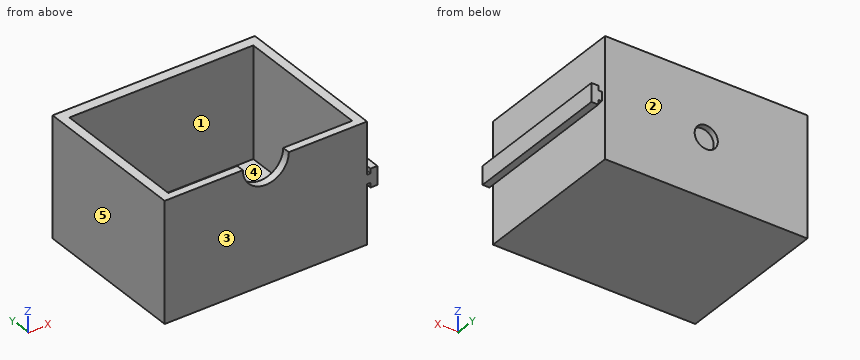
from build123d import *

# Parameters (mm, degrees)
F0_W     = 55.88
F0_H     = 33.02
F1_DEPTH = 43.18
F2_W     = 50.8
F2_H     = 38.1
F3_DEPTH = 30.48
F4_R     = 6.35
F5_DEPTH = 25.4
F6_R     = 3.2
F7_DEPTH = 1.6002
F9_DEPTH = 41.91


with BuildPart() as f1:
    # F0 (on Front) → F1 (new body)
    with BuildSketch(Plane.XZ):
        with Locations((-20.484024, 16.51)):
            Rectangle(F0_W, F0_H)
    extrude(amount=-F1_DEPTH)

    # F2 (on face) → F3 (cut)
    with BuildSketch(Plane.XY.offset(33.02)):
        with Locations((-20.484024, 21.216264)):
            Rectangle(F2_W, F2_H)
    extrude(amount=-F3_DEPTH, mode=Mode.SUBTRACT)

    # F4 (on face) → F5 (cut)
    with BuildSketch(Plane.XZ):
        with Locations((-20.484024, 33.02)):
            Circle(F4_R)
    extrude(amount=-F5_DEPTH, mode=Mode.SUBTRACT)

    # F6 (on face) → F7 (cut)
    with BuildSketch(Plane(origin=(0, 43.18, 0), x_dir=(-1, 0, 0), z_dir=(0, 1, 0))):
        with Locations((20.484024, 16.51)):
            Circle(F6_R)
    extrude(amount=-F7_DEPTH, mode=Mode.SUBTRACT)

    # F8 (on face) → F9 (join)
    with BuildSketch(Plane.XZ):
        Polygon((8.421195, 20.018721), (8.421195, 18.748721), (7.455976, 18.748721), (7.455976, 16.208721), (8.421195, 16.208721), (8.421195, 14.938721), (10.326195, 14.938721), (10.326195, 20.018721), align=None)
    extrude(amount=-F9_DEPTH)


solid = f1.part
The listing builds one solid part. Answer for the finished solid, in the listing's coordinates (mm). Face numbers are marked on the shaded views. A direction names the side the tool comes from. Round coordinates to 2 decimals unless told otherwise and drop trailing zeros. Order: outer loops, then holes, each group sorted by start corner. A loop starts at its lowest first (then second) coordinate and runs counter-clockwise, first axis right, second up. Notation, with made-up numbers: (9.5, -22) - (65.5, -22) arc R25 cw to (65.5, -1) - close; hole circle Ø11 at (-19.75, -21). An arc over 180 degrees is marked (long way). Write item = value, one per line. Start each with the question number.
1) Straight lines are drawn through the part: L1, parallel to Y at x = -9.5, z = 23; L2, parallel to X at y = 23, z = 22.5; L3, parallel to Z at x = -5, y = 22. For each, find the intervals that lie inside material, in ascending order.
2) Given pin 1 (4 mm diameter, centred on x = -20.48, z = 16.51, fed in from +Y); pin 2 (10 mm diameter, centred on x = -21, z = 29.5, fed in from -Y); pin 3 (1.5 mm diameter, centred on x = 9, y = 17.5, fed in from +Z); pin 4 (5 mm diameter, centred on y = 32, z = 11, fed in from +X), each flat-ended and moving along its own axis, determine where each tip first touches the part or whether it passes through.
3) Section D-D, the plane z = 28 is taken. Write down the section's boundary in (x, y), plus the area to 3 significant figures.
4) For the marked faces 1 and 2, determine the directions among +Z, -Z, +X, -X, +Y, -Y from which every point of the face is accessible in a straight line to the end or side of a thin tool.
5) For a pull along X with two mould halves and no side action, classify the marked faces 3, 4 and 5 as released by +X, released by -X, zero draft, split by the parting line, or undercut.
6) Section A-A, the plane z = 8.5 is taken. Write down the section's boundary in (x, y).
7) Section C-C, the plane y = 16 is taken. Write down the section's boundary in (x, z).
8) Section B-B, the plane x = -2 is taken. Write down the section's boundary in (y, z), plus the area to 3 significant figures.
Results list:
q1.L1 = 0 to 2.17, 40.27 to 43.18
q1.L2 = -48.42 to -45.88, 4.92 to 7.46
q1.L3 = 0 to 2.54
q2.pin_1 = 41.58
q2.pin_2 = 0
q2.pin_3 = 20.02
q2.pin_4 = 7.46
q3.outline = (-48.42, 0) - (-24.37, 0) - (-24.37, 2.17) - (-45.88, 2.17) - (-45.88, 40.27) - (4.92, 40.27) - (4.92, 2.17) - (-16.6, 2.17) - (-16.6, 0) - (7.46, 0) - (7.46, 43.18) - (-48.42, 43.18) - close
q3.area = 461 mm^2
q4.face_1 = +Z
q4.face_2 = +Z, -Z, +X, -X, +Y
q5.face_3 = zero draft
q5.face_4 = undercut
q5.face_5 = released by -X
q6.outline = (-48.42, 0) - (7.46, 0) - (7.46, 43.18) - (-48.42, 43.18) - close; hole (-45.88, 2.17) - (4.92, 2.17) - (4.92, 40.27) - (-45.88, 40.27) - close
q7.outline = (-48.42, 0) - (7.46, 0) - (7.46, 16.21) - (8.42, 16.21) - (8.42, 14.94) - (10.33, 14.94) - (10.33, 20.02) - (8.42, 20.02) - (8.42, 18.75) - (7.46, 18.75) - (7.46, 33.02) - (4.92, 33.02) - (4.92, 2.54) - (-45.88, 2.54) - (-45.88, 33.02) - (-48.42, 33.02) - close
q8.outline = (0, 0) - (43.18, 0) - (43.18, 33.02) - (40.27, 33.02) - (40.27, 2.54) - (2.17, 2.54) - (2.17, 33.02) - (0, 33.02) - close
q8.area = 265 mm^2
